Here's how the part is built. I have some questions about the finished solid (model axes, mm). A direction names the side the tool comes from. Give positions to 0.01 mm unless a question says otherwise; leave off trailing zeros. Loops run counter-clockwise (first coordinate to the right, second up) from the corner with the lowest first, then second, coordinate; pieces in that order, holes last. Notation, with made-up numbers: (-28.75, 21) - (25.25, 21) arc R4 ccw to (25.25, 26) - close; hole circle Ø4 at (23.5, 38). An arc over 180 degrees is marked (long way). Return JSON: item names as keys, results as strings. Group by question number.
(1) For P1, Ø5.5, axis at x = -14.94, y = 8.62, coming from the -Z side; P2, Ø8, axis at x = 14.5, z = 11.5, coming from the +Y side; P3, Ø9.5, axis at x = 0, y = 42.5, coming from the -Z side; P4, Ø6.5, axis at x = 14.94, y = 8.62, coming from the +Z side, each with a flat end and sliding along its axis, tell me the tip position at first contact or that it passes through.
(2) If we section it at C-C (z = 3): Please give me the cut outline in (x, y) (3 decimals), then the cut area to 3 significant figures.
(3) On a 3-axis mill with a long thin cutter (end or side, diameter ignored), from which of +Z, -Z, +X, -X, +Y, -Y can I reach the whole of each face in a straight line? I mean faces 1 (the cylindrical face through (1.94, 16.45, 8.21)), 2 (the cylindrical face through (33.05, -29.92, 13.77)). Say none if no direction works.
(4) If we section it at B-B (x = -42.5): Please give me the cut outline in (y, z), then the cut area to 3 significant figures.
(5) I need wall thicknesses on probe 1 along X at (y, z) = (-7, 7.5); probe 2 along X at (y, z) = (9, 6.5); probe 3 along Y at (x, z) = (42.5, 14.3). Which ranges of each line are inside material? Lowest first, please. Write a range as [from, to].
(6) If we section it at D-D (z = 17.75): State how many separate pieces and enclosed holes the cut face has, then the cut area to 3 significant figures.
(7) If we section it at A-A (y = 0): Please give me the cut outline in (x, z).
(8) If we mould it in two halves opening along X, with no side actions, what happens to faces 3 (the flat face through (1, -1, 19.6)), 4 (the cylindrical face through (-46.022, -14.493, 15.747)), 5 (the cylindrical face through (-27.055, -29.92, 13.775))? For each: released by +X, released by -X, zero draft, split by the parting line, or undercut.
```python
from build123d import *

# Parameters (mm, degrees)
SKETCH_1_R               = 29.5
EXTRUDE_1_DEPTH          = 12
SKETCH_2_R               = 48.25
EXTRUDE_2_DEPTH          = 7.6
FILLET_1_R               = 5
SKETCH_4_R               = 3
CUT_EXTRUDE_1_DEPTH      = 3.6
SKETCH_5_R               = 2.1
CUT_EXTRUDE_2_DEPTH      = 45.6
PATTERN_CIRCULAR_1_COUNT = 6
SKETCH_7_R               = 1.8
CUT_EXTRUDE_3_DEPTH      = 45.6


with BuildPart() as part:
    # Sketch 1 → Extrude 1 (new body)
    with BuildSketch(Plane.XY):
        Circle(SKETCH_1_R)
    extrude(amount=EXTRUDE_1_DEPTH)

    # Sketch 2 → Extrude 2 (add)
    with BuildSketch(Plane.XY.offset(12)):
        with Locations(Location((0, 0, 0), (0, 0, 180))):
            Circle(SKETCH_2_R)
    extrude(amount=EXTRUDE_2_DEPTH)

    # Fillet 1
    fillet_1_edges = [part.edges().sort_by_distance(p)[0] for p in [
        (-29.5, 0, 12),
    ]]
    fillet(fillet_1_edges, radius=FILLET_1_R)

    # Sketch 4 → Cut-Extrude 1 (cut)
    with BuildSketch(Plane(origin=(0, 0, 12), x_dir=(-1, 0, 0), z_dir=(0, 0, -1))):
        with Locations((0, 42.5)):
            Circle(SKETCH_4_R)
        with Locations((30.0520382, 30.0520382)):
            Circle(SKETCH_4_R)
        with Locations((42.5, 0)):
            Circle(SKETCH_4_R)
        with Locations((30.0520382, -30.0520382)):
            Circle(SKETCH_4_R)
        with Locations((0, -42.5)):
            Circle(SKETCH_4_R)
        with Locations((-30.0520382, -30.0520382)):
            Circle(SKETCH_4_R)
        with Locations((-42.5, 0)):
            Circle(SKETCH_4_R)
        with Locations((-30.0520382, 30.0520382)):
            Circle(SKETCH_4_R)
    extrude(amount=-CUT_EXTRUDE_1_DEPTH, mode=Mode.SUBTRACT)

    # Sketch 5 → Cut-Extrude 2 (cut)
    with BuildSketch(Plane.XY.offset(19.6)):
        with Locations((0, 17.25)):
            Circle(SKETCH_5_R)
        with Locations((14.938938215, 8.625)):
            Circle(SKETCH_5_R)
        with Locations((14.938938215, -8.625)):
            Circle(SKETCH_5_R)
        with Locations((0, -17.25)):
            Circle(SKETCH_5_R)
        with Locations((-14.938938215, -8.625)):
            Circle(SKETCH_5_R)
        with Locations((-14.938938215, 8.625)):
            Circle(SKETCH_5_R)
    extrude(amount=-CUT_EXTRUDE_2_DEPTH, mode=Mode.SUBTRACT)

    # Sketch 6 → Cut-Revolve 1 (revolve, cut)
    with BuildSketch(Plane(origin=(7.469469108, 12.9375, 0), x_dir=(0.8660254037844382, -0.500000000000001, 0), z_dir=(0.5000000000000009, 0.866025403784438, 0)), mode=Mode.PRIVATE) as cut_revolve_1_sk:
        Polygon((8.625, -16.2), (8.625, -19.6), (10.725, -19.6), (12.625, -19.6), (10.725, -16.2), align=None)
    cut_revolve_1 = revolve(cut_revolve_1_sk.sketch.rotate(Axis((14.938938215, 8.625, 0), (0, 0, 1)), 30), axis=Axis((14.938938215, 8.625, 0), (0, 0, 1)), mode=Mode.SUBTRACT)

    # Pattern Circular 1: Cut-Revolve 1 ×6 about axis
    pattern_circular_1_axis = Axis((0, 0, 0), (0, 0, 1))
    for i in range(1, PATTERN_CIRCULAR_1_COUNT):
        add(cut_revolve_1.rotate(pattern_circular_1_axis, i * 360 / PATTERN_CIRCULAR_1_COUNT), mode=Mode.SUBTRACT)

    # Sketch 7 → Cut-Extrude 3 (cut)
    with BuildSketch(Plane(origin=(0, 0, 15.6), x_dir=(-1, 0, 0), z_dir=(0, 0, -1))):
        with Locations((0, 42.5)):
            Circle(SKETCH_7_R)
        with Locations((-30.0520382, 30.0520382)):
            Circle(SKETCH_7_R)
        with Locations((-42.5, 0)):
            Circle(SKETCH_7_R)
        with Locations((-30.0520382, -30.0520382)):
            Circle(SKETCH_7_R)
        with Locations((0, -42.5)):
            Circle(SKETCH_7_R)
        with Locations((30.0520382, -30.0520382)):
            Circle(SKETCH_7_R)
        with Locations((42.5, 0)):
            Circle(SKETCH_7_R)
        with Locations((30.0520382, 30.0520382)):
            Circle(SKETCH_7_R)
    extrude(amount=-CUT_EXTRUDE_3_DEPTH, mode=Mode.SUBTRACT)


solid = part.part
```
Values:
{
 "1": {"P1": "z = 0", "P2": "y = 47.09", "P3": "z = 12", "P4": "z = 18.27"},
 "2": {"outline": "circle Ø59 at (0, 0); hole circle Ø4.2 at (-14.939, -8.625); hole circle Ø4.2 at (-14.939, 8.625); hole circle Ø4.2 at (0, -17.25); hole circle Ø4.2 at (0, 17.25); hole circle Ø4.2 at (14.939, -8.625); hole circle Ø4.2 at (14.939, 8.625)", "area": "2,650 mm2"},
 "3": {"face 1": "+Z, -Z", "face 2": "-Z"},
 "4": {"outline": "(-22.84, 12) - (-3, 12) - (-3, 15.6) - (-1.8, 15.6) - (-1.8, 19.6) - (-22.84, 19.6) - close; (1.8, 15.6) - (3, 15.6) - (3, 12) - (22.84, 12) - (22.84, 19.6) - (1.8, 19.6) - close", "area": "311 mm2"},
 "5": {"probe 1": "[-28.68, -16.27], [-13.61, 13.61], [16.27, 28.68]", "probe 2": "[-28.09, -17.01], [-12.87, 12.87], [17.01, 28.09]", "probe 3": "[-22.84, -3], [3, 22.84]"},
 "6": {"separate pieces": "1", "enclosed holes": "14", "area": "7,070 mm2"},
 "7": {"outline": "(-48.25, 12) - (-45.5, 12) - (-45.5, 15.6) - (-44.3, 15.6) - (-44.3, 19.6) - (-48.25, 19.6) - close; (-40.7, 15.6) - (-39.5, 15.6) - (-39.5, 12) - (-34.5, 12) arc R5 cw to (-29.5, 7) - (-29.5, 0) - (29.5, 0) - (29.5, 7) arc R5 cw to (34.5, 12) - (39.5, 12) - (39.5, 15.6) - (40.7, 15.6) - (40.7, 19.6) - (-40.7, 19.6) - close; (44.3, 15.6) - (45.5, 15.6) - (45.5, 12) - (48.25, 12) - (48.25, 19.6) - (44.3, 19.6) - close"},
 "8": {"face 3": "zero draft", "face 4": "split by the parting line", "face 5": "undercut"}
}
